Geometry: final body of the model. Coordinates: model frame, mm. A direction names the side the tool comes from. Give positions to 0.01 mm unless a question says otherwise; leave off trailing zeros. Order: outer loops, then holes, each group sorted by start corner. A loop starts at its lowest first (then second) coordinate and runs counter-clockwise, first axis right, second up. Notation, with made-up numbers: (-22, 25) -> (2, 25) arc R8 ccw to (2, 36) -> close; hole circle Ø1 at (57.25, 76). An arc over 180 degrees is marked (long way). One line per item, written item: value. Start each with the question number.
Autodesk Inventor part; units mm, degrees
ref_plane "Start plane" through (0, 0, 0) normal (0, 0, 1) x (1, 0, 0)
ref_plane "End plane" through (0, 0, 651) normal (0, 0, 1) x (1, 0, 0)
ref_plane "Work Plane5" through (0, 15, 651) normal (0, -0.7071, 0.7071) x (1, 0, 0)
ref_plane "Start plane" through (0, 0, 0) normal (0, 0, 1) x (1, 0, 0)
ref_plane "End plane" through (0, 0, 651) normal (0, 0, 1) x (1, 0, 0)
sketch "Sketch" plane through (0, 0, 0) normal (0, 0, 1) x (1, 0, 0)
  line L0 (-15, -11.25) -> (-15, 11.25)
  line L1 (-11.25, 15) -> (11.25, 15)
  line L2 (15, 11.25) -> (15, -11.25)
  line L3 (11.25, -15) -> (-11.25, -15)
  arc A0 (-15, -11.25) -> (-11.25, -15) centre (-11.25, -11.25) ccw
  arc A1 (-11.25, 15) -> (-15, 11.25) centre (-11.25, 11.25) ccw
  arc A2 (15, 11.25) -> (11.25, 15) centre (11.25, 11.25) ccw
  arc A3 (11.25, -15) -> (15, -11.25) centre (11.25, -11.25) ccw
  arc A4 (-11.25, 12.5) -> (-12.5, 11.25) centre (-11.25, 11.25) ccw
  line L4 (-11.25, 12.5) -> (11.25, 12.5)
  arc A5 (12.5, 11.25) -> (11.25, 12.5) centre (11.25, 11.25) ccw
  line L5 (12.5, 11.25) -> (12.5, -11.25)
  arc A6 (11.25, -12.5) -> (12.5, -11.25) centre (11.25, -11.25) ccw
  line L6 (11.25, -12.5) -> (-11.25, -12.5)
  arc A7 (-12.5, -11.25) -> (-11.25, -12.5) centre (-11.25, -11.25) ccw
  line L7 (-12.5, -11.25) -> (-12.5, 11.25)
  line L8 (0, 22.0873) -> (0, -22.0873) construction
  line L9 (-22.0873, 0) -> (22.0873, 0) construction
  dimension "d7" = 3.75
  dimension "d10" = 30
  dimension "d11" = 30
  dimension "d12" = 2.5
  dimension "d15" = 15
  dimension "d16" = 15
extrude "Body" add sketch "Sketch" along normal up to surface (651 mm away) from surface at 0
sketch "Sketch3" plane through (0, 0, 0) normal (0, 0, 1) x (1, 0, 0)
  line L0 (0, 0) -> (10, 0)
ref_plane "Work Plane3" through (0, 0, 0) normal (0, -1, 0) x (1, 0, 0)
sketch "Sketch4" plane through (0, 0, 0) normal (0, -1, 0) x (1, 0, 0)
  line L0 (-2, 0) -> (12, 0)
  line L1 (-2, 651) -> (12, 651)
  dimension "d18" = 651
ref_plane "Work Plane5" through (0, 15, 651) normal (0, -0.7071, 0.7071) x (1, 0, 0)
split "Split2" plane through (0, 15, 651) removes the side toward (0, -0.7071, 0.7071)
ref_plane "Work Plane6" through (0, 15, 0) normal (0, -0.7071, -0.7071) x (1, 0, 0)
split "Split3" plane through (0, 15, 0) removes the side toward (0, -0.7071, -0.7071)
equation "\"d7\" = G_IR"
equation "\"d10\" = G_H"
equation "\"d11\" = G_W"
equation "\"d12\" = G_T"
equation "\"d15\" = 0.5 * d10"
equation "\"d16\" = 0.5 * d11"
equation "\"d3\" = G_L"
equation "\"G_W\" = 30"
equation "\"G_H\" = 30"
equation "\"G_T\" = 2.5"
equation "\"G_IR\" = 3.75"
equation "\"G_L\" = d18"
equation "\"G_OFFSET_START\" = 0"
equation "\"G_OFFSET_END\" = 0"
equation "\"d14\" = G_OFFSET_END + B_L"
equation "\"B_L\" = 651"
properties part number "DIN EN 10305-5 - 30 x 30 x 2,5  - 651" material "Steel, Mild"
1. Access query for faces 4 (the flat face through (0, -12.5, 321)), 5 (the flat face through (15, 0, 321)). Directions: +Z, -Z, +X, -X, +Y, -Y. A direction counts if a zero-diameter tool reaches every point of the face in a straight line with its end or side. Return the directions, or none.
2. Cut plane B-B, the plane x = -0.75. Return loops of the section in (y, z), then the cut area to 4 significant figures.
3. Pin query (flat end, axial travel): P1, Ø5, axis at x = -4, y = 8.5, coming from the +Z side; P2, Ø3, axis at x = -12, y = 10.5, coming from the +Z side. Return the tip coordinate at first contact, or that it passes through.
4. Material intervals for L1, parallel to Y at x = 2.25, z = 202.5; L2, parallel to X at y = -12, z = 108, sorted ascending. Write a range as [from, to].
5. Draft query along X for faces 1 (the flat face through (0, -15, 321)), 2 (the flat face through (0, 12.5, 321)), 3 (the flat face through (-15, 0, 321)). Return one class per face: pulls with the +X half, pulls with the -X half, needs draft (parallel to the pull), parting line crosses it, or undercut.
6. Cut plane A-A, the plane y = -1.5. Return loops of the section in (x, z).
7. Cut plane C-C, the plane z = 288. Return loops of the section in (x, y), then the cut area to 3 significant figures.
Answers follow:
1. face 4: +Z, -Z
1. face 5: +Z, -Z, +X, +Y, -Y
2. outline: (-15, 30) -> (-12.5, 27.5) -> (-12.5, 623.5) -> (-15, 621) -> close; (12.5, 2.5) -> (15, 0) -> (15, 651) -> (12.5, 648.5) -> close
2. area: 3,105 mm²
3. P1: passes through
3. P2: stops at z = 647.98
4. L1: y = [-15, -12.5], [12.5, 15]
4. L2: x = [-14.92, -12.25], [12.25, 14.92]
5. face 1: needs draft
5. face 2: undercut
5. face 3: pulls with the -X half
6. outline: (-15, 16.5) -> (-12.5, 16.5) -> (-12.5, 634.5) -> (-15, 634.5) -> close; (12.5, 16.5) -> (15, 16.5) -> (15, 634.5) -> (12.5, 634.5) -> close
7. outline: (-15, -11.25) arc R3.75 ccw to (-11.25, -15) -> (11.25, -15) arc R3.75 ccw to (15, -11.25) -> (15, 11.25) arc R3.75 ccw to (11.25, 15) -> (-11.25, 15) arc R3.75 ccw to (-15, 11.25) -> close; hole (-12.5, -11.25) arc R1.25 ccw to (-11.25, -12.5) -> (11.25, -12.5) arc R1.25 ccw to (12.5, -11.25) -> (12.5, 11.25) arc R1.25 ccw to (11.25, 12.5) -> (-11.25, 12.5) arc R1.25 ccw to (-12.5, 11.25) -> close
7. area: 264 mm²
